from build123d import *

# Parameters (mm, degrees)
SKETCH_1_W      = 65
SKETCH_1_H      = 5
EXTRUDE_2_DEPTH = 30
SKETCH_4_W      = 10
SKETCH_4_H      = 5
EXTRUDE_4_DEPTH = 30


with BuildPart() as part:
    # 스케치1 → 보스-돌출2 (new body)
    # profile 1 of 2: a face of its own
    with BuildSketch(Plane.XY):
        with Locations((27.5, 21.5)):
            Rectangle(SKETCH_1_W, SKETCH_1_H)
    # profile 2 of 2: a face of its own
    with BuildSketch(Plane.XY):
        Polygon((-5, 19), (-5, -5), (7, -5), (7, 7), (60, 7), (60, 19), align=None)
        Polygon((2, 0), (0, 0), (0, 14), (10, 14), (10, 18), (52, 18), (52, 14), (55, 14), (55, 12), (2, 12), align=None, mode=Mode.SUBTRACT)
    extrude(amount=EXTRUDE_2_DEPTH)

    # 스케치4 → 보스-돌출4 (add)
    with BuildSketch(Plane(origin=(0, 0, 0), x_dir=(-1, 0, 0), z_dir=(0, 0, -1))):
        Polygon((93, 19), (5, 19), (5, -5), (93, -5), (93, 14), align=None)
        with Locations((98, 16.5)):
            Rectangle(SKETCH_4_W, SKETCH_4_H)
    extrude(amount=-EXTRUDE_4_DEPTH)


solid = part.part
Build history of the part. All positions in model axes, mm. A direction names the side the tool comes from. Round coordinates to 2 decimals unless told otherwise and drop trailing zeros. Write each loop counter-clockwise with the first axis right and the second up, starting at its lowest first coordinate (ties: lowest second). Pieces come first, ordered by that corner, then holes. Notation, with made-up numbers: (85, 51) -> (116, 51) arc R10 ccw to (116, 60) -> close; hole circle Ø10 at (16, -4). An arc over 180 degrees is marked (long way). Write item = value, one per line.
(1) Band-saw the part on D-D (y = -2.75). Give the cut face in (x, z), then the cut area to 3 significant figures.
Answer:
outline = (-93, 0) -> (7, 0) -> (7, 30) -> (-93, 30) -> close
area = 3,000 mm2
(2) Band-saw the part on A-A (y = 9.25). Give the cut face in (x, z).
Answer:
outline = (-93, 0) -> (0, 0) -> (0, 30) -> (-93, 30) -> close; (2, 0) -> (60, 0) -> (60, 30) -> (2, 30) -> close
(3) Tool access for faces 1 (the face through (0, 7, 15)), 2 (the face through (-5, 22, 15)), 3 (the face through (-93, 4, 15)), 4 (the face through (7, 1, 15)), 5 (the face through (60, 15, 15)): list every direction of +Z, -Z, +X, -X, +Y, -Y with a clear straight run to the whole face (end or side of a thin tool).
Answer:
face_1 = +Z, -Z
face_2 = +Z, -Z, -X, +Y
face_3 = +Z, -Z, -X, -Y
face_4 = +Z, -Z, +X, -Y
face_5 = +Z, -Z, +X, +Y, -Y
(4) Probe L1, parallel to Y at x = 6, z = 18; L2, parallel to Y at x = 45, z = 28.5; L3, parallel to X at y = 16.5, z = 18.25. List the from-to ranges inside material, lowest first.
Answer:
L1 = -5 to 12, 14 to 24
L2 = 7 to 12, 18 to 24
L3 = -103 to 10, 52 to 60
(5) Two-plate mould, pull along X, no slides. Class faces 6 (the face through (31, 18, 15)), 7 (the face through (-103, 16, 15)), 8 (the face through (-98, 14, 15)): pulls with the +X half, pulls with the -X half, needs draft (parallel to the pull), parting line crosses it, or undercut.
Answer:
face_6 = undercut
face_7 = pulls with the -X half
face_8 = needs draft
(6) Band-saw the part on C-C (z = 15). Give the cut face in (x, y).
Answer:
outline = (-103, 14) -> (-93, 14) -> (-93, -5) -> (7, -5) -> (7, 7) -> (60, 7) -> (60, 24) -> (-5, 24) -> (-5, 19) -> (-103, 19) -> close; hole (0, 0) -> (2, 0) -> (2, 12) -> (55, 12) -> (55, 14) -> (52, 14) -> (52, 18) -> (10, 18) -> (10, 14) -> (0, 14) -> close
(7) Band-saw the part on B-B (x = 17.5). Give the cut face in (y, z).
Answer:
outline = (7, 0) -> (12, 0) -> (12, 30) -> (7, 30) -> close; (18, 0) -> (24, 0) -> (24, 30) -> (18, 30) -> close
(8) Flat gauge pins, fed straight in: pin 1 (3.5 mm diameter, centred on y = 3.5, z = 19, fed in from +X); pin 2 (15 mm diameter, centred on x = -50.5, z = 9, fed in from +Y); pin 3 (5 mm diameter, centred on x = -50.5, y = 21, fed in from -Z); pin 4 (15 mm diameter, centred on x = 42, z = 12, fed in from -Y). Where does each tip first touch, or does it go through?
Answer:
pin_1 = 7
pin_2 = 19
pin_3 = 0
pin_4 = 7
